```python
from build123d import *

# Parameters (mm, degrees)
SKETCH_W     = 10
SKETCH_H     = 10
PAD_DEPTH    = 10
SKETCH001_R  = 4.75
PAD001_DEPTH = 10
FILLET_R     = 4.45


with BuildPart() as part:
    # Sketch → Pad (new body)
    with BuildSketch(Plane.XY):
        Rectangle(SKETCH_W, SKETCH_H)
    extrude(amount=PAD_DEPTH)

    # Sketch001 (on Face6 of Pad) → Pad001 (join)
    with BuildSketch(Plane.XY.offset(10)):
        Circle(SKETCH001_R)
    extrude(amount=PAD001_DEPTH)

    # Fillet
    fillet_edges = [part.edges().sort_by_distance(p)[0] for p in [
        (-4.75, 0, 20),
    ]]
    fillet(fillet_edges, radius=FILLET_R)


solid = part.part
```
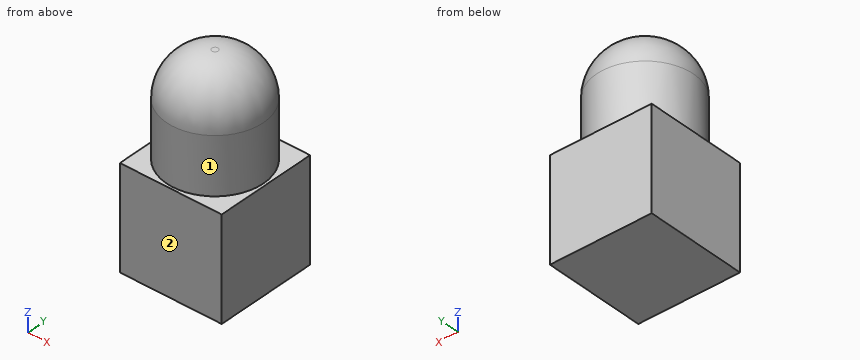
The listing builds one solid part. Answer for the finished solid, in the listing's coordinates (mm). Face numbers are marked on the shaded views. A direction names the side the tool comes from. Round coordinates to 2 decimals unless told otherwise and drop trailing zeros. Loops run counter-clockwise (first coordinate to the right, second up) from the corner with the lowest first, then second, coordinate; pieces in that order, holes last. Notation, with made-up numbers: (76.25, -15) - (126.25, -15) arc R13 cw to (126.25, -4) - close; hole circle Ø8 at (-14, -8). An arc over 180 degrees is marked (long way). Return JSON: item names as keys, results as strings. Group by question number.
1. Each of these flat-tipped pins is pushed along its axis until it touches: P1, Ø3, axis at x = -3, y = 4, coming from the +Z side; P2, Ø1.5, axis at y = -2, z = 11.5, coming from the -X side; P3, Ø2, axis at y = 3.5, z = 16, coming from the +X side. Where does it stop, or does it pass through?
2. Consider probe 1 along Z at (x, y) = (3.25, 3.5); probe 2 along Y at (x, z) = (0, 11.5); probe 3 along Y at (x, z) = (2, 17.25). Determine where each line is inside the solid, lowest interval first.
3. The part is cut by section A-A on z = 14.5. Determine the outline of the cut face in (x, y).
4. Which of the six approach directions +Z, -Z, +X, -X, +Y, -Y give full straight-line access (tool end or side, diameter ignored) to the marked faces 1 and 2?
Resolved:
{
 "1": {"P1": "stops at z = 18.64", "P2": "stops at x = -4.58", "P3": "stops at x = 4.02"},
 "2": {"probe 1": "z = 0 to 10", "probe 2": "y = -4.75 to 4.75", "probe 3": "y = -3.93 to 3.93"},
 "3": {"outline": "circle Ø9.5 at (0, 0)"},
 "4": {"face 1": "+Z", "face 2": "+Z, -Z, +X, -X, -Y"}
}
